Build history of the part. All positions in model axes, mm. Give positions to 0.01 mm unless a question says otherwise; leave off trailing zeros. Order: outer loops, then holes, each group sorted by start corner. A loop starts at its lowest first (then second) coordinate and runs counter-clockwise, first axis right, second up. Notation, with made-up numbers: (65.25, 75) - (115.25, 75) arc R20 cw to (115.25, 90) - close; hole circle Ø1 at (40, 69.5). An arc over 180 degrees is marked (long way). Use a Markdown table: item, result. Add a question column.
(1) Slice it at A-A (x = 8). Write the cut outline in (y, z), then the cut area to 3 significant figures.
(2) Wall check: line 1 (Z direction, x = 74, y = 2.95); line 2 (X direction, y = 1.6, z = -53); line 3 (X direction, y = 0.85, z = -48.5). Give the ranges that are in metal, low to high.
(3) Slice it at B-B (z = -53). Write the cut outline in (x, y), then the cut area to 3 significant figures.
(4) Slice it at C-C (y = 0.95). Write the cut outline in (x, z).
(5) Slice it at D-D (z = -44.5). Write the cut outline in (x, y).
(6) Flat gauge pins, fed straight in: pin 1 (2 mm diameter, centred on y = 2.5, z = -22, fed in from +X); pin 2 (2 mm diameter, centred on y = 3, z = -22.5, fed in from -X). Where does each tip first touch, or does it go through?
from build123d import *

# Parameters (mm, degrees)
SKETCH1_R           = 1.8
BOSS_EXTRUDE1_DEPTH = 4
SKETCH2_W           = 29.307012988
SKETCH2_H           = 22
SKETCH2_W_2         = 22
SKETCH2_H_2         = 29.307012987
CUT_EXTRUDE1_DEPTH  = 103.279030109
FILLET1_R           = 10


with BuildPart() as part:
    # Sketch1 → Boss-Extrude1 (new body)
    with BuildSketch(Plane(origin=(0, 0, 0), x_dir=(1, 0, 0), z_dir=(0, 1, 0))):
        with BuildLine():
            Line((0, 0), (82, 0))
            Line((82, 0), (82, 56))
            ThreePointArc((82, 56), (80.535533906, 59.535533906), (77, 61))
            Line((77, 61), (5, 61))
            ThreePointArc((5, 61), (1.464466094, 59.535533906), (0, 56))
            Line((0, 56), (0, 0))
        make_face()
        with Locations(Location((8, 53, 0), (0, 0, 270))):
            Circle(SKETCH1_R, mode=Mode.SUBTRACT)
        with Locations(Location((74, 53, 0), (0, 0, 270))):
            Circle(SKETCH1_R, mode=Mode.SUBTRACT)
    extrude(amount=BOSS_EXTRUDE1_DEPTH)

    # Sketch2 → Cut-Extrude1 (cut, through all)
    with BuildSketch(Plane(origin=(0, 4, 0), x_dir=(1, 0, 0), z_dir=(0, 1, 0))):
        with Locations((41, 50)):
            Rectangle(SKETCH2_W, SKETCH2_H)
        with Locations((71, 20.653506494)):
            Rectangle(SKETCH2_W_2, SKETCH2_H_2)
        with Locations((11, 20.653506494)):
            Rectangle(SKETCH2_W_2, SKETCH2_H_2)
    extrude(amount=-CUT_EXTRUDE1_DEPTH, mode=Mode.SUBTRACT)

    # Fillet1
    fillet1_edges = [part.edges().sort_by_distance(p)[0] for p in [
        (26.346493506, 2, -39),
        (55.653506494, 2, -39),
        (60, 2, -6),
        (60, 2, -35.307012987),
        (22, 2, -35.307012987),
        (22, 2, -6),
    ]]
    fillet(fillet1_edges, radius=FILLET1_R)


solid = part.part
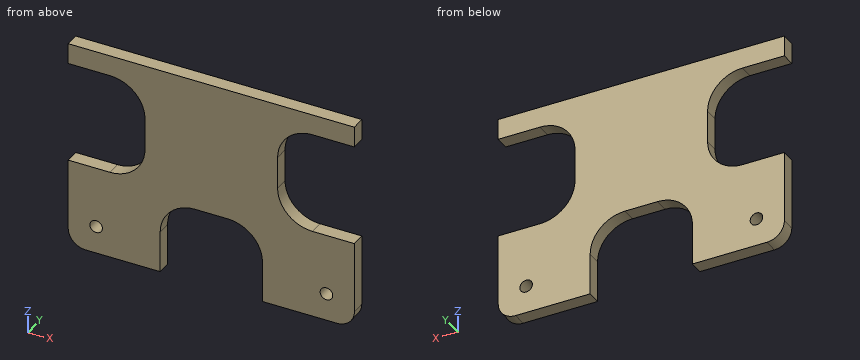
Solution:
| question | item | result |
|---|---|---|
| 1 | outline | (0, -61) - (4, -61) - (4, -54.8) - (0, -54.8) - close; (0, -51.2) - (4, -51.2) - (4, -35.31) - (0, -35.31) - close; (0, -6) - (4, -6) - (4, 0) - (0, 0) - close |
| 1 | area | 112 mm2 |
| 2 | line 1 | -61 to -54.8, -51.2 to -35.31, -6 to 0 |
| 2 | line 2 | 0 to 6.2, 9.8 to 26.35, 55.65 to 72.2, 75.8 to 82 |
| 2 | line 3 | 0 to 26.36, 55.64 to 82 |
| 3 | outline | (0, 0) - (6.2, 0) - (6.2, 4) - (0, 4) - close; (9.8, 0) - (26.35, 0) - (26.35, 4) - (9.8, 4) - close; (55.65, 0) - (72.2, 0) - (72.2, 4) - (55.65, 4) - close; (75.8, 0) - (82, 0) - (82, 4) - (75.8, 4) - close |
| 3 | area | 182 mm2 |
| 4 | outline | (0, -56) arc R5 ccw to (5, -61) - (26.35, -61) - (26.35, -49) arc R10 cw to (36.35, -39) - (45.65, -39) arc R10 cw to (55.65, -49) - (55.65, -61) - (77, -61) arc R5 ccw to (82, -56) - (82, -35.31) - (70, -35.31) arc R10 cw to (60, -25.31) - (60, -16) arc R10 cw to (70, -6) - (82, -6) - (82, 0) - (0, 0) - (0, -6) - (12, -6) arc R10 cw to (22, -16) - (22, -25.31) arc R10 cw to (12, -35.31) - (0, -35.31) - close; hole circle Ø3.6 at (8, -53); hole circle Ø3.6 at (74, -53) |
| 5 | outline | (0, 0) - (27.42, 0) - (27.42, 4) - (0, 4) - close; (54.58, 0) - (82, 0) - (82, 4) - (54.58, 4) - close |
| 6 | pin 1 | x = 60 |
| 6 | pin 2 | x = 22 |
